from build123d import *

# Parameters (mm, degrees)
BOSS_EXTRUDE1_DEPTH      = 120
BOSS_EXTRUDE1_DEPTH_BACK = 120
CUT_EXTRUDE1_START       = -17
SKETCH2_R                = 4
CUT_EXTRUDE1_DEPTH       = 18
SKETCH3_R                = 4
CUT_EXTRUDE2_DEPTH       = 1
CUT_EXTRUDE2_DEPTH_BACK  = 17


with BuildPart() as part:
    # Sketch1 → Boss-Extrude1 (new body, two sides)
    with BuildSketch(Plane.XY) as boss_extrude1_sk:
        with BuildLine():
            Line((-6, -8), (6, -8))
            ThreePointArc((6, -8), (7.414213562, -7.414213562), (8, -6))
            Line((8, -6), (8, 6))
            ThreePointArc((8, 6), (7.414213562, 7.414213562), (6, 8))
            Line((6, 8), (-6, 8))
            ThreePointArc((-6, 8), (-7.414213562, 7.414213562), (-8, 6))
            Line((-8, 6), (-8, -6))
            ThreePointArc((-8, -6), (-7.414213562, -7.414213562), (-6, -8))
        make_face()
        with BuildLine():
            Line((-6, 7.32), (6, 7.32))
            ThreePointArc((6, 7.32), (6.933380951, 6.933380951), (7.32, 6))
            Line((7.32, 6), (7.32, -6))
            ThreePointArc((7.32, -6), (6.933380951, -6.933380951), (6, -7.32))
            Line((6, -7.32), (-6, -7.32))
            ThreePointArc((-6, -7.32), (-6.933380951, -6.933380951), (-7.32, -6))
            Line((-7.32, -6), (-7.32, 6))
            ThreePointArc((-7.32, 6), (-6.933380951, 6.933380951), (-6, 7.32))
        make_face(mode=Mode.SUBTRACT)
    extrude(amount=BOSS_EXTRUDE1_DEPTH)
    extrude(boss_extrude1_sk.sketch, amount=-BOSS_EXTRUDE1_DEPTH_BACK)

    # Sketch2 → Cut-Extrude1 (cut)
    with BuildSketch(Plane(origin=(0, 8, 0), x_dir=(1, 0, 0), z_dir=(0, 1, 0)).offset(CUT_EXTRUDE1_START)):
        with Locations((0, -50)):
            Circle(SKETCH2_R)
    cut_extrude1 = extrude(amount=CUT_EXTRUDE1_DEPTH, mode=Mode.SUBTRACT)

    # Mirror1: Cut-Extrude1 across plane
    add(cut_extrude1.mirror(Plane.XY), mode=Mode.SUBTRACT)

    # Sketch3 → Cut-Extrude2 (cut, two sides)
    with BuildSketch(Plane(origin=(8, 0, 0), x_dir=(0, 0, -1), z_dir=(1, 0, 0))) as cut_extrude2_sk:
        with Locations((-100, 0)):
            Circle(SKETCH3_R)
        with Locations((100, 0)):
            Circle(SKETCH3_R)
    extrude(amount=CUT_EXTRUDE2_DEPTH, mode=Mode.SUBTRACT)
    extrude(cut_extrude2_sk.sketch, amount=-CUT_EXTRUDE2_DEPTH_BACK, mode=Mode.SUBTRACT)


solid = part.part
Can you work these out from the model? Positions are in its coordinate system, mm. A direction names the side the tool comes from. Coordinates: 2 decimals unless noted, no trailing zeros. Loops run counter-clockwise (first coordinate to the right, second up) from the corner with the lowest first, then second, coordinate; pieces in that order, holes last. Notation, with made-up numbers: M -30,-34.75 L 25,-34.75 A7 cw 25,-28.75 Z; hole C -11,28.25 d6. An arc over 180 degrees is marked long. Answer as CSV lines item,"result". Start each with the question number.
1. If I drill on probe 1 along Z at (x, y) = (0, -7.6); probe 2 along X at (y, z) = (2.25, 96), over which ranges is the centre line in solid material (lowest first)? Write a range as [from, to].
2. Suppose I cut it at A-A, the plane x = 0. List the corners of the cut face in (y, z) for me, plus the area to 3 significant figures.
3. For faces 5 (the face through (7.32, 0, 2)), 6 (the face through (0, -7.7, -120)), which set-ups out of +Z, -Z, +X, -X, +Y, -Y let a thin tool reach every point of the face, with its end or its side?
4. Suppose I cut it at C-C, the plane z = -50. List the corners of the cut face in (x, y) for me.
5. Thinking about a two-plate mould opening in Y: for faces 1 (the face through (7.665, -1.532, -103.695)), 2 (the face through (7.665, 0.176, 103.996)), 3 (the face through (1.846, -7.665, -53.549)), 4 (the face through (0, 8, 2)), which applies, +Y half, -Y half, draft (parallel to the pull), parting line (faces both ways), or undercut?
6. Suppose I cut it at B-B, the plane y = 0. List the corners of the cut face in (x, z) for me.
7. Suppose I cut it at D-D, the plane z = 98. List the corners of the cut face in (x, y) for me.
Output:
1,probe 1,"z = [-120, -54], [-46, 46], [54, 120]"
1,probe 2,"x = [-8, -7.32], [7.32, 8]"
2,outline,"M -8,-120 L -7.32,-120 L -7.32,-54 L -8,-54 Z; M -8,-46 L -7.32,-46 L -7.32,46 L -8,46 Z; M -8,54 L -7.32,54 L -7.32,120 L -8,120 Z; M 7.32,-120 L 8,-120 L 8,-54 L 7.32,-54 Z; M 7.32,-46 L 8,-46 L 8,46 L 7.32,46 Z; M 7.32,54 L 8,54 L 8,120 L 7.32,120 Z"
2,area,"305 mm^2"
3,face 5,"+Z, -Z"
3,face 6,"-Z, +X, -X, +Y, -Y"
4,outline,"M -8,-6 A2 ccw -6,-8 L -4,-8 L -4,-7.32 L -6,-7.32 A1.32 cw -7.32,-6 L -7.32,6 A1.32 cw -6,7.32 L -4,7.32 L -4,8 L -6,8 A2 ccw -8,6 Z; M 4,-8 L 6,-8 A2 ccw 8,-6 L 8,6 A2 ccw 6,8 L 4,8 L 4,7.32 L 6,7.32 A1.32 cw 7.32,6 L 7.32,-6 A1.32 cw 6,-7.32 L 4,-7.32 Z"
5,face 1,"undercut"
5,face 2,"undercut"
5,face 3,"draft"
5,face 4,"+Y half"
6,outline,"M -8,-120 L -7.32,-120 L -7.32,-104 L -8,-104 Z; M -8,-96 L -7.32,-96 L -7.32,96 L -8,96 Z; M -8,104 L -7.32,104 L -7.32,120 L -8,120 Z; M 7.32,-120 L 8,-120 L 8,-104 L 7.32,-104 Z; M 7.32,-96 L 8,-96 L 8,96 L 7.32,96 Z; M 7.32,104 L 8,104 L 8,120 L 7.32,120 Z"
7,outline,"M -8,-6 A2 ccw -6,-8 L 6,-8 A2 ccw 8,-6 L 8,-3.46 L 7.32,-3.46 L 7.32,-6 A1.32 cw 6,-7.32 L -6,-7.32 A1.32 cw -7.32,-6 L -7.32,-3.46 L -8,-3.46 Z; M -8,3.46 L -7.32,3.46 L -7.32,6 A1.32 cw -6,7.32 L 6,7.32 A1.32 cw 7.32,6 L 7.32,3.46 L 8,3.46 L 8,6 A2 ccw 6,8 L -6,8 A2 ccw -8,6 Z"
